Can you work these out from the model? Positions are in its coordinate system, mm. A direction names the side the tool comes from. Give positions to 0.01 mm unless a question says otherwise; leave off trailing zeros. Loops run counter-clockwise (first coordinate to the right, second up) from the corner with the lowest first, then second, coordinate; pieces in that order, holes last. Notation, with made-up numbers: M 36.25,89 L 45.25,89 A11 ccw 45.25,96 Z; hole C 77.25,10.25 d11. An arc over 180 degrees is marked long. Use CSV: the item, a comma, the result in double quotes.
from build123d import *

# Parameters (mm, degrees)
SKETCH2_R           = 23.5
SKETCH2_R_2         = 1
BOSS_EXTRUDE1_DEPTH = 3
FILLET1_R           = 5
SKETCH3_R           = 1
CUT_EXTRUDE1_DEPTH  = 3
CIRPATTERN1_COUNT   = 3


with BuildPart() as part:
    # Sketch2 → Boss-Extrude1 (new body)
    with BuildSketch(Plane(origin=(0, 0, 0), x_dir=(1, 0, 0), z_dir=(0, 1, 0))):
        with BuildLine():
            Line((24.819347292, 15), (54.819347292, 15))
            Line((54.819347292, 15), (62.319347292, 22.5))
            Line((62.319347292, 22.5), (76.319347292, 22.5))
            Line((76.319347292, 22.5), (76.319347292, -22.5))
            Line((76.319347292, -22.5), (62.319347292, -22.5))
            Line((62.319347292, -22.5), (54.819347292, -15))
            Line((54.819347292, -15), (24.819347292, -15))
            ThreePointArc((24.819347292, -15), (-29, 0), (24.819347292, 15))
        make_face()
        with Locations(Location((0, 0, 0), (0, 0, 270))):
            Circle(SKETCH2_R, mode=Mode.SUBTRACT)
        with Locations(Location((72.319347292, 10, 0), (0, 0, 270))):
            Circle(SKETCH2_R_2, mode=Mode.SUBTRACT)
        with Locations(Location((72.319347292, -10, 0), (0, 0, 270))):
            Circle(SKETCH2_R_2, mode=Mode.SUBTRACT)
    extrude(amount=BOSS_EXTRUDE1_DEPTH)

    # Fillet1
    fillet1_edges = [part.edges().sort_by_distance(p)[0] for p in [
        (54.819347292, 1.5, -15),
        (62.319347292, 1.5, -22.5),
        (62.319347292, 1.5, 22.5),
        (54.819347292, 1.5, 15),
        (24.819347292, 1.5, 15),
        (24.819347292, 1.5, -15),
    ]]
    fillet(fillet1_edges, radius=FILLET1_R)

    # Sketch3 → Cut-Extrude1 (cut)
    with BuildSketch(Plane(origin=(0, 3, 0), x_dir=(1, 0, 0), z_dir=(0, 1, 0))):
        with Locations(Location((13.25, 22.9496732, 0), (0, 0, 270))):
            Circle(SKETCH3_R)
    cut_extrude1 = extrude(amount=-CUT_EXTRUDE1_DEPTH, mode=Mode.SUBTRACT)

    # CirPattern1: Cut-Extrude1 ×3 about axis
    cirpattern1_axis = Axis((0, 0, 0), (0, 1, 0))
    for i in range(1, CIRPATTERN1_COUNT):
        add(cut_extrude1.rotate(cirpattern1_axis, i * 360 / CIRPATTERN1_COUNT), mode=Mode.SUBTRACT)


solid = part.part
Q1. I'm going to push flat-ended pins straight in: P1, Ø1, axis at x = 58, y = 1.5, coming from the -Z side; P2, Ø1.5, axis at x = 45.5, y = 1, coming from the +Z side; P3, Ø1.5, axis at x = 68.5, y = 1.5, coming from the +Z side. Where does each tip first touch, or does it pass through?
Model answer:
P1,"z = -18.68"
P2,"z = 15"
P3,"z = 22.5"
Q2. I want a section at B-B, the plane z = -2. Please give me the cut outline in (x, y).
Model answer:
outline,"M -28.93,0 L -23.41,0 L -23.41,3 L -28.93,3 Z; M 23.41,0 L 76.32,0 L 76.32,3 L 23.41,3 Z"
Q3. Please list where these lines run through material, in increasing order: L1, parallel to X at y = 1.1, z = 0; L2, parallel to X at y = 0.6, z = 18; L3, parallel to Z at x = -9, y = 2.45. Write a range as from..to.
Model answer:
L1,"-29..-27.5, -25.5..-23.5, 23.5..76.32"
L2,"-22.74..-15.11, 15.11..22.74, 57.82..76.32"
L3,"-27.57..-21.71, 21.71..27.57"
Q4. I want a section at C-C, the plane z = 10. Please give me the cut outline in (x, y), then the cut area to 3 significant figures.
Model answer:
outline,"M -27.22,0 L -21.27,0 L -21.27,3 L -27.22,3 Z; M 21.27,0 L 71.32,0 L 71.32,3 L 21.27,3 Z; M 73.32,0 L 76.32,0 L 76.32,3 L 73.32,3 Z"
area,"177 mm2"
Q5. I want a section at D-D, the plane y = 0.8. Please give me the cut outline in (x, z).
Model answer:
outline,"M 23.45,-17.06 A5 cw 27.5,-15 L 52.75,-15 A5 cw 56.28,-16.46 L 60.85,-21.04 A5 ccw 64.39,-22.5 L 76.32,-22.5 L 76.32,22.5 L 64.39,22.5 A5 ccw 60.85,21.04 L 56.28,16.46 A5 cw 52.75,15 L 27.5,15 A5 cw 23.45,17.06 A29 ccw long Z; hole C -26.5,0 d2; hole C 0,0 d47; hole C 13.25,-22.95 d2; hole C 13.25,22.95 d2; hole C 72.32,-10 d2; hole C 72.32,10 d2"
Q6. If we mould it in two halves opening along X, with no side actions, what happens to faces 4 (the flat face through (36, 3, 0)), 5 (the flat face through (76.319, 1, 0)), 6 (the flat face through (40, 1, -15)), 7 (the cylindrical face through (14.09, 1.52, 23.49))? For each: released by +X, released by -X, zero draft, split by the parting line, or undercut.
Model answer:
face 4,"zero draft"
face 5,"released by +X"
face 6,"undercut"
face 7,"undercut"
Q7. I want a section at A-A, the plane x = 0. Please give me the cut outline in (y, z).
Model answer:
outline,"M 0,-29 L 3,-29 L 3,-23.5 L 0,-23.5 Z; M 0,23.5 L 3,23.5 L 3,29 L 0,29 Z"
Q8. For faces 1 (the flat face through (70, 1, -22.5)), 2 (the cylindrical face through (62.45, 1.52, 22.11)), 3 (the cylindrical face through (25.256, 1.521, -15.529)), which set-ups out of +Z, -Z, +X, -X, +Y, -Y let a thin tool reach every point of the face, with its end or its side?
Model answer:
face 1,"-Z, +X, +Y, -Y"
face 2,"+Z, +Y, -Y"
face 3,"-Z, +Y, -Y"
